from build123d import *

# Parameters (mm, degrees)
SKETCH3_R                   = 101.6
BOSS_EXTRUDE1_DEPTH         = 6.35
SKETCH4_R                   = 6.35
CUT_EXTRUDE1_DEPTH          = 144.824345992
F_10_32_TAPPED_HOLE1_D      = 4.0386
F_10_32_TAPPED_HOLE1_DEPTH  = 13.716
F_10_32_TAPPED_HOLE1_TIP    = 1.213317848
SKETCH6_W                   = 63.5
SKETCH6_H                   = 25.4
SKETCH6_R                   = 12.7
CUT_EXTRUDE2_DEPTH          = 3.175
F_1_4_20_TAPPED_HOLE2_D     = 5.1054
F_1_4_20_TAPPED_HOLE2_DEPTH = 19.05
F_1_4_20_TAPPED_HOLE2_TIP   = 1.533816902
F_1_4_20_TAPPED_HOLE4_D     = 5.1054
F_1_4_20_TAPPED_HOLE4_DEPTH = 19.05
F_1_4_20_TAPPED_HOLE4_TIP   = 1.533816902


with BuildPart() as part:
    # Sketch3 → Boss-Extrude1 (new body)
    with BuildSketch(Plane(origin=(0, 0, 0), x_dir=(1, 0, 0), z_dir=(0, 1, 0))):
        with Locations(Location((0, 0, 0), (0, 0, 270))):
            Circle(SKETCH3_R)
    extrude(amount=BOSS_EXTRUDE1_DEPTH)

    # Sketch4 → Cut-Extrude1 (cut, through all)
    with BuildSketch(Plane(origin=(0, 6.35, 0), x_dir=(1, 0, 0), z_dir=(0, 1, 0))):
        with BuildLine():
            ThreePointArc((0, -6.35), (4.490128061, -4.490128061), (6.35, 0))
            Line((6.35, 0), (0, 0))
            Line((0, 0), (0, -6.35))
        make_face()
        with BuildLine():
            Line((0, 0), (6.35, 0))
            ThreePointArc((6.35, 0), (-4.490128061, 4.490128061), (0, -6.35))
            Line((0, -6.35), (0, 0))
        make_face()
        with Locations(Location((26.662380423, -26.662380423, 0), (0, 0, 270))):
            Circle(SKETCH4_R)
    extrude(amount=-CUT_EXTRUDE1_DEPTH, mode=Mode.SUBTRACT)

    # #10-32 Tapped Hole1
    with Locations(Plane(origin=(0, 6.35, -85.599778), x_dir=(0, 0, 1), z_dir=(0, 1, 0))):
        with Locations((0, 0), (85.599778, -85.599778), (171.199556, 0), (85.599778, 85.599778)):
            Hole(F_10_32_TAPPED_HOLE1_D / 2, depth=F_10_32_TAPPED_HOLE1_DEPTH)
            with Locations((0, 0, -(F_10_32_TAPPED_HOLE1_DEPTH + F_10_32_TAPPED_HOLE1_TIP / 2))):  # 118° drill point
                Cone(0, F_10_32_TAPPED_HOLE1_D / 2, F_10_32_TAPPED_HOLE1_TIP, mode=Mode.SUBTRACT)

    # Sketch6 → Cut-Extrude2 (cut)
    # profile 1 of 4: a face of its own
    with BuildSketch(Plane(origin=(0, 6.35, 0), x_dir=(1, 0, 0), z_dir=(0, 1, 0))):
        with BuildLine():
            Line((-28.575, 61.9125), (-6.35, 61.9125))
            Line((-6.35, 61.9125), (-6.35, 95.038097624))
            ThreePointArc((-6.35, 95.038097624), (-67.351920908, 67.351920908), (-95.038097624, 6.35))
            Line((-95.038097624, 6.35), (-10.998522628, 6.35))
            ThreePointArc((-10.998522628, 6.35), (-8.980256121, 8.980256121), (-6.35, 10.998522628))
            Line((-6.35, 10.998522628), (-6.35, 39.6875))
            Line((-6.35, 39.6875), (-28.575, 39.6875))
            Line((-28.575, 39.6875), (-28.575, 61.9125))
        make_face()
    # profile 2 of 4: a face of its own
    with BuildSketch(Plane(origin=(0, 6.35, 0), x_dir=(1, 0, 0), z_dir=(0, 1, 0))):
        with BuildLine():
            Line((6.35, 95.038097624), (6.35, 61.9125))
            Line((6.35, 61.9125), (28.575, 61.9125))
            Line((28.575, 61.9125), (28.575, 39.6875))
            Line((28.575, 39.6875), (6.35, 39.6875))
            Line((6.35, 39.6875), (6.35, 10.998522628))
            ThreePointArc((6.35, 10.998522628), (8.980256121, 8.980256121), (10.998522628, 6.35))
            Line((10.998522628, 6.35), (95.038097624, 6.35))
            ThreePointArc((95.038097624, 6.35), (67.351920908, 67.351920908), (6.35, 95.038097624))
        make_face()
    # profile 3 of 4: a face of its own
    with BuildSketch(Plane(origin=(0, 6.35, 0), x_dir=(1, 0, 0), z_dir=(0, 1, 0))):
        with BuildLine():
            ThreePointArc((-6.35, -10.998522628), (-8.980256121, -8.980256121), (-10.998522628, -6.35))
            Line((-10.998522628, -6.35), (-95.038097624, -6.35))
            ThreePointArc((-95.038097624, -6.35), (-67.351920908, -67.351920908), (-6.35, -95.038097624))
            Line((-6.35, -95.038097624), (-6.35, -10.998522628))
        make_face()
        with Locations((-40.4114, -38.1)):
            Rectangle(SKETCH6_W, SKETCH6_H, mode=Mode.SUBTRACT)
    # profile 4 of 4: a face of its own
    with BuildSketch(Plane(origin=(0, 6.35, 0), x_dir=(1, 0, 0), z_dir=(0, 1, 0))):
        with BuildLine():
            Line((95.038097624, -6.35), (10.998522628, -6.35))
            ThreePointArc((10.998522628, -6.35), (8.980256121, -8.980256121), (6.35, -10.998522628))
            Line((6.35, -10.998522628), (6.35, -95.038097624))
            ThreePointArc((6.35, -95.038097624), (67.351920908, -67.351920908), (95.038097624, -6.35))
        make_face()
        with Locations(Location((26.662380423, -26.662380423, 0), (0, 0, 270))):
            Circle(SKETCH6_R, mode=Mode.SUBTRACT)
    extrude(amount=-CUT_EXTRUDE2_DEPTH, mode=Mode.SUBTRACT)

    # 1/4-20 Tapped Hole2
    with Locations(Plane(origin=(-22.225, 6.35, -50.8), x_dir=(0, 0, 1), z_dir=(0, 1, 0))):
        with Locations((0, 0), (0, 44.45), (0, 22.225)):
            Hole(F_1_4_20_TAPPED_HOLE2_D / 2, depth=F_1_4_20_TAPPED_HOLE2_DEPTH)
            with Locations((0, 0, -(F_1_4_20_TAPPED_HOLE2_DEPTH + F_1_4_20_TAPPED_HOLE2_TIP / 2))):  # 118° drill point
                Cone(0, F_1_4_20_TAPPED_HOLE2_D / 2, F_1_4_20_TAPPED_HOLE2_TIP, mode=Mode.SUBTRACT)

    # 1/4-20 Tapped Hole4
    with Locations(Plane(origin=(-65.8114, 6.35, 31.75), x_dir=(0, 0, 1), z_dir=(0, 1, 0))):
        with Locations((0, 0), (12.7, 0), (12.7, 50.8), (0, 50.8)):
            Hole(F_1_4_20_TAPPED_HOLE4_D / 2, depth=F_1_4_20_TAPPED_HOLE4_DEPTH)
            with Locations((0, 0, -(F_1_4_20_TAPPED_HOLE4_DEPTH + F_1_4_20_TAPPED_HOLE4_TIP / 2))):  # 118° drill point
                Cone(0, F_1_4_20_TAPPED_HOLE4_D / 2, F_1_4_20_TAPPED_HOLE4_TIP, mode=Mode.SUBTRACT)


solid = part.part
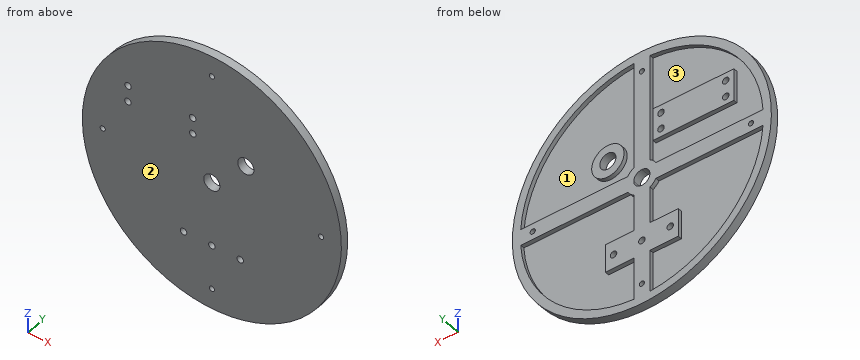
Source: CAD feature listing. Evaluate the final solid. Frame: model axes, mm. Face numbers are marked on the shaded views. Round coordinates to 2 decimals unless told otherwise and drop trailing zeros. Loops run counter-clockwise (first coordinate to the right, second up) from the corner with the lowest first, then second, coordinate; pieces in that order, holes last. Notation, with made-up numbers: M 47,44 L 76,44 A30 cw 76,72 Z; hole C 41.25,38.25 d3. An arc over 180 degrees is marked long. Return JSON: item names as keys, results as strings. Group by question number.
1. Section query C-C on x = -35.5. Output: boundary loops of the cut face in (y, z) (3 decimals), and give its area (3 significant figures).
2. Material intervals for line 1 along Z through (x, y) = (77.5, 3.75); line 2 along Z through (x, y) = (-85.5, 4.5); line 3 along X through (y, z) = (3, 31.75), sorted ascending. Write a range as from..to.
3. Pin query (flat end, axial travel): pin 1 (1.6 mm diameter, centred on y = 5, z = -75.5, fed in from -X); pin 2 (1 mm diameter, centred on x = 64, y = 2.5, fed in from -Z); pin 3 (1.5 mm diameter, centred on x = -5.5, y = 3.5, fed in from +Z); pin 4 (3.5 mm diameter, centred on x = 85.6, z = 0, fed in from -Y). Return the tip coordinate at first contact, or that it passes through.
4. Mould query, pull axis X, two halves, no side actions, for the marked faces 1, 2 and 3. Classes: released by +X, released by -X, zero draft, split by the parting line, or undercut.
5. Section query B-B on z = 44.45. Output: boundary loops of the cut face in (x, y) (3 decimals), and give its area (3 significant figures).
6. Section query A-A on z = -50.8. Output: boundary loops of the cut face in (x, y) (3 decimals).
Checks:
{
 "1": {"outline": "M 0,-95.196 L 6.35,-95.196 L 6.35,-88.387 L 3.175,-88.387 L 3.175,-6.35 L 6.35,-6.35 L 6.35,6.35 L 3.175,6.35 L 3.175,25.4 L 6.35,25.4 L 6.35,50.8 L 3.175,50.8 L 3.175,88.387 L 6.35,88.387 L 6.35,95.196 L 0,95.196 Z", "area": "769 mm²"},
 "2": {"line 1": "z = -65.7..-55.37, -6.35..6.35, 55.37..65.7", "line 2": "z = -54.88..-41.98, -6.35..-2.02, 2.02..6.35, 41.98..54.88", "line 3": "x = -96.51..-68.36, -63.26..-17.56, -12.46..22.86, 30.46..96.51"},
 "3": {"pin 1": "stops at x = -68.87", "pin 2": "stops at z = -79.31", "pin 3": "stops at z = 101.49", "pin 4": "passes through"},
 "4": {"face 1": "undercut", "face 2": "zero draft", "face 3": "undercut"},
 "5": {"outline": "M -91.361,0 L -68.364,0 L -68.364,6.35 L -72.161,6.35 L -72.161,3.175 L -84.242,3.175 L -84.242,6.35 L -91.361,6.35 Z; M -63.259,0 L -17.564,0 L -17.564,6.35 L -63.259,6.35 Z; M -12.459,0 L 91.361,0 L 91.361,6.35 L 84.242,6.35 L 84.242,3.175 L 6.35,3.175 L 6.35,6.35 L -6.35,6.35 L -6.35,3.175 L -8.661,3.175 L -8.661,6.35 L -12.459,6.35 Z", "area": "802 mm²"},
 "6": {"outline": "M -87.988,0 L -24.778,0 L -24.778,6.35 L -28.575,6.35 L -28.575,3.175 L -80.572,3.175 L -80.572,6.35 L -87.988,6.35 Z; M -19.672,0 L -2.553,0 L -2.553,6.35 L -19.672,6.35 Z; M 2.553,0 L 19.672,0 L 19.672,6.35 L 2.553,6.35 Z; M 24.778,0 L 87.988,0 L 87.988,6.35 L 80.572,6.35 L 80.572,3.175 L 28.575,3.175 L 28.575,6.35 L 24.778,6.35 Z"}
}
